The model under review builds one solid part; all positions refer to its coordinate system, in mm. Face numbers are marked on the shaded views. Give positions to 0.01 mm unless a question says otherwise; leave off trailing zeros. Loops run counter-clockwise (first coordinate to the right, second up) from the corner with the lowest first, then second, coordinate; pieces in that order, holes last. Notation, with made-up numbers: (52.5, -33.75) - (100.5, -33.75) arc R16 cw to (100.5, -21.75) - close; hole circle Ø4 at (0.5, 21). An arc over 180 degrees is marked (long way). Answer as a JSON object with one key per item and string values.
from build123d import *

# Parameters (mm, degrees)
SKETCH1_R           = 29.35
SKETCH1_R_2         = 27.5
BOSS_EXTRUDE1_DEPTH = 60
BOSS_EXTRUDE2_DEPTH = 6
FILLET1_R           = 2
FILLET2_R           = 0.5
BOSS_EXTRUDE3_REACH = 93.389
SKETCH3_R           = 14
SKETCH3_R_2         = 11.5
BOSS_EXTRUDE4_START = 11
SKETCH3_3_R         = 14
SKETCH3_3_R_2       = 11.5
BOSS_EXTRUDE4_DEPTH = 11
BOSS_EXTRUDE5_START = 4
SKETCH4_R           = 14.125
SKETCH4_R_2         = 11.5
BOSS_EXTRUDE5_DEPTH = 4
BOSS_EXTRUDE6_START = 4
SKETCH5_R           = 14.25
SKETCH5_R_2         = 11.5
BOSS_EXTRUDE6_DEPTH = 4
BOSS_EXTRUDE7_START = 4
SKETCH6_R           = 14.375
SKETCH6_R_2         = 11.5
BOSS_EXTRUDE7_DEPTH = 4
BOSS_EXTRUDE8_START = 4
SKETCH7_R           = 14.5
SKETCH7_R_2         = 11.5
BOSS_EXTRUDE8_DEPTH = 4
FILLET3_R           = 2
CUT_EXTRUDE1_REACH  = 112.683
SKETCH8_R           = 11.5
BOSS_EXTRUDE9_START = -0.5
SKETCH9_R           = 27.5
BOSS_EXTRUDE9_DEPTH = 0.5


with BuildPart() as part:
    # Sketch1 → Boss-Extrude1 (new body)
    with BuildSketch(Plane.XY):
        Circle(SKETCH1_R)
        Circle(SKETCH1_R_2, mode=Mode.SUBTRACT)
    extrude(amount=BOSS_EXTRUDE1_DEPTH)

    # Sketch2 → Boss-Extrude2 (add)
    with BuildSketch(Plane.XY.offset(33.3)):
        with BuildLine():
            Line((-28.503026155, 7), (-36.143026155, 7))
            Line((-36.143026155, 7), (-36.143026155, -7))
            Line((-36.143026155, -7), (-28.503026155, -7))
            ThreePointArc((-28.503026155, -7), (-28.729407073, -6.003638001), (-28.920969901, -5))
            Line((-28.920969901, -5), (-34.143026155, -5))
            Line((-34.143026155, -5), (-34.143026155, 5))
            Line((-34.143026155, 5), (-28.920969901, 5))
            ThreePointArc((-28.920969901, 5), (-28.729407073, 6.003638001), (-28.503026155, 7))
        make_face()
        with BuildLine():
            Line((28.503026155, 7), (36.143026155, 7))
            Line((36.143026155, 7), (36.143026155, -7))
            Line((36.143026155, -7), (28.503026155, -7))
            ThreePointArc((28.503026155, -7), (28.729407073, -6.003638001), (28.920969901, -5))
            Line((28.920969901, -5), (34.143026155, -5))
            Line((34.143026155, -5), (34.143026155, 5))
            Line((34.143026155, 5), (28.920969901, 5))
            ThreePointArc((28.920969901, 5), (28.729407073, 6.003638001), (28.503026155, 7))
        make_face()
    extrude(amount=BOSS_EXTRUDE2_DEPTH)

    # Fillet1
    fillet1_edges = [part.edges().sort_by_distance(p)[0] for p in [
        (-28.503026155, 7, 36.3),
        (-36.143026155, 7, 36.3),
        (-36.143026155, -7, 36.3),
        (-28.503026155, -7, 36.3),
        (28.503026155, -7, 36.3),
        (36.143026155, -7, 36.3),
        (36.143026155, 7, 36.3),
        (28.503026155, 7, 36.3),
    ]]
    fillet(fillet1_edges, radius=FILLET1_R)

    # Fillet2
    fillet2_edges = [part.edges().sort_by_distance(p)[0] for p in [
        (-29.35, 0, 60),
    ]]
    fillet(fillet2_edges, radius=FILLET2_R)

    # Sketch3 → Boss-Extrude3 (add, up to next)
    with BuildSketch(Plane(origin=(0, -29.35, 0), x_dir=(-1, 0, 0), z_dir=(0, -1, 0)), mode=Mode.PRIVATE) as boss_extrude3_sk1:
        with Locations((12.85, -16.5)):
            Circle(SKETCH3_R)
        with Locations(Location((12.85, -16.5, 0), (0, 0, 90))):
            Circle(SKETCH3_R_2, mode=Mode.SUBTRACT)
    boss_extrude3_tool1 = extrude(boss_extrude3_sk1.sketch, amount=-BOSS_EXTRUDE3_REACH, mode=Mode.PRIVATE) - part.part
    add(boss_extrude3_tool1.solids().sort_by_distance((0.75402, -29.35, 16.5))[0])
    add(boss_extrude3_tool1.solids().sort_by_distance((0.75402, -29.35, 16.5))[1])

    # Sketch3<3> → Boss-Extrude4 (add)
    with BuildSketch(Plane(origin=(0, -29.35, 0), x_dir=(-1, 0, 0), z_dir=(0, -1, 0)).offset(BOSS_EXTRUDE4_START)):
        with Locations(Location((12.85, -16.5, 0), (0, 0, 90))):
            Circle(SKETCH3_3_R)
        with Locations(Location((12.85, -16.5, 0), (0, 0, 90))):
            Circle(SKETCH3_3_R_2, mode=Mode.SUBTRACT)
    extrude(amount=-BOSS_EXTRUDE4_DEPTH)

    # Sketch4 → Boss-Extrude5 (add)
    with BuildSketch(Plane(origin=(0, -40.35, 0), x_dir=(-1, 0, 0), z_dir=(0, -1, 0)).offset(BOSS_EXTRUDE5_START)):
        with Locations(Location((12.85, -16.5, 0), (0, 0, 90))):
            Circle(SKETCH4_R)
        with Locations(Location((12.85, -16.5, 0), (0, 0, 90))):
            Circle(SKETCH4_R_2, mode=Mode.SUBTRACT)
    extrude(amount=-BOSS_EXTRUDE5_DEPTH)

    # Sketch5 → Boss-Extrude6 (add)
    with BuildSketch(Plane.XZ.offset(44.35).offset(BOSS_EXTRUDE6_START)):
        with Locations(Location((-12.85, 16.5, 0), (0, 0, 270))):
            Circle(SKETCH5_R)
        with Locations(Location((-12.85, 16.5, 0), (0, 0, 270))):
            Circle(SKETCH5_R_2, mode=Mode.SUBTRACT)
    extrude(amount=-BOSS_EXTRUDE6_DEPTH)

    # Sketch6 → Boss-Extrude7 (add)
    with BuildSketch(Plane.XZ.offset(48.35).offset(BOSS_EXTRUDE7_START)):
        with Locations(Location((-12.85, 16.5, 0), (0, 0, 270))):
            Circle(SKETCH6_R)
        with Locations(Location((-12.85, 16.5, 0), (0, 0, 270))):
            Circle(SKETCH6_R_2, mode=Mode.SUBTRACT)
    extrude(amount=-BOSS_EXTRUDE7_DEPTH)

    # Sketch7 → Boss-Extrude8 (add)
    with BuildSketch(Plane(origin=(0, -52.35, 0), x_dir=(-1, 0, 0), z_dir=(0, -1, 0)).offset(BOSS_EXTRUDE8_START)):
        with Locations(Location((12.85, -16.5, 0), (0, 0, 90))):
            Circle(SKETCH7_R)
        with Locations(Location((12.85, -16.5, 0), (0, 0, 90))):
            Circle(SKETCH7_R_2, mode=Mode.SUBTRACT)
    extrude(amount=-BOSS_EXTRUDE8_DEPTH)

    # Fillet3
    fillet3_edges = [part.edges().sort_by_distance(p)[0] for p in [
        (-12.85, -56.35, 31),
    ]]
    fillet(fillet3_edges, radius=FILLET3_R)

    # Sketch8 → Cut-Extrude1 (cut, up to next)
    with BuildSketch(Plane.XZ.offset(56.35), mode=Mode.PRIVATE) as cut_extrude1_sk1:
        with Locations(Location((-12.85, 16.5, 0), (0, 0, 270))):
            Circle(SKETCH8_R)
    cut_extrude1_tool1 = extrude(cut_extrude1_sk1.sketch, amount=-CUT_EXTRUDE1_REACH, mode=Mode.PRIVATE) & part.part
    add(cut_extrude1_tool1.solids().sort_by_distance((-12.85, -56.35, 16.5))[0], mode=Mode.SUBTRACT)

    # Sketch9 → Boss-Extrude9 (add)
    with BuildSketch(Plane.XY.offset(60).offset(BOSS_EXTRUDE9_START)):
        Circle(SKETCH9_R)
    extrude(amount=BOSS_EXTRUDE9_DEPTH)


solid = part.part
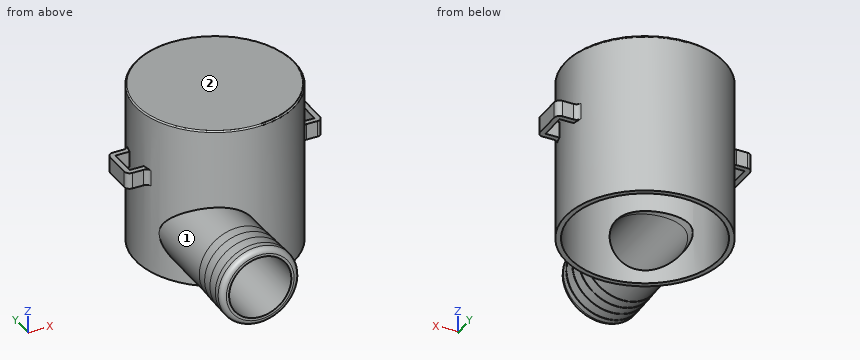
Q1. To check wall thickness, follow probe 1 along Z at (x, y) = (-12.85, -25.5); probe 2 along Z at (x, y) = (-12.85, -29); probe 3 along Y at (x, z) = (-22, 45.5). State the ranges of each line that lie inside material, in increasing order. Write a range as [from, to].
Results:
{"probe 1": "z = [0, 5], [28, 60]", "probe 2": "z = [2.5, 5], [28, 30.5]", "probe 3": "y = [-19.43, -16.5], [16.5, 19.43]"}
Q2. Consider section A-A, the plane z = 37. State the section outline as (x, y) points, plus the area to 3 significant figures.
Results:
{"outline": "(-36.14, -5) arc R2 ccw to (-34.14, -7) - (-30.03, -7) arc R2 cw to (-28.11, -8.43) arc R29.35 ccw to (28.11, -8.43) arc R2 cw to (30.03, -7) - (34.14, -7) arc R2 ccw to (36.14, -5) - (36.14, 5) arc R2 ccw to (34.14, 7) - (30.03, 7) arc R2 cw to (28.11, 8.43) arc R29.35 ccw to (-28.11, 8.43) arc R2 cw to (-30.03, 7) - (-34.14, 7) arc R2 ccw to (-36.14, 5) - close; hole (-34.14, -5) - (-28.92, -5) arc R29.35 cw to (-28.92, 5) - (-34.14, 5) - close; hole circle Ø55 at (0, 0); hole (28.92, -5) - (34.14, -5) - (34.14, 5) - (28.92, 5) arc R29.35 cw to start", "area": "428 mm^2"}
Q3. Consider section C-C, the plane y = -43. State the section outline as (x, z) points (3 decimals), plus the area to 3 significant figures.
Results:
{"outline": "circle Ø28.25 at (-12.85, 16.5); hole circle Ø23 at (-12.85, 16.5)", "area": "211 mm^2"}
Q4. Consider section B-B, the plane y = 0. State the section outline as (x, z) points.
Results:
{"outline": "(-36.14, 33.3) - (-34.14, 33.3) - (-34.14, 39.3) - (-36.14, 39.3) - close; (-29.35, 0) - (-27.5, 0) - (-27.5, 59.5) - (27.5, 59.5) - (27.5, 0) - (29.35, 0) - (29.35, 59.5) arc R0.5 ccw to (28.85, 60) - (-28.85, 60) arc R0.5 ccw to (-29.35, 59.5) - close; (34.14, 33.3) - (36.14, 33.3) - (36.14, 39.3) - (34.14, 39.3) - close"}
Q5. The part is to be moulded in two halves that separate along Y. For the marked faces 1 and 2, say which applies: +Y half, -Y half, draft (parallel to the pull), parting line (faces both ways), or undercut.
Results:
{"face 1": "undercut", "face 2": "draft"}
Q6. Clearance check with flat-ended pins moving along their axes: pin 1 Ø2.5 at (x, y) = (-33.5, -3.5) entering from -Z; pin 2 Ø4.5 at (x, z) = (31.5, 36.5) entering from -Y; pin 3 Ø6 at (x, z) = (-14.5, 12) entering from -Y. State where each tip first meets the part, or that it passes through.
Results:
{"pin 1": "stops at z = 33.3", "pin 2": "stops at y = -7.16", "pin 3": "stops at y = 21.21"}
Q7. Consider section D-D, the plane z = 54.5. State the section outline as (x, y) points.
Results:
{"outline": "circle Ø58.7 at (0, 0); hole circle Ø55 at (0, 0)"}
